CAD build for the part. Positions are in the model's coordinates, mm. A direction names the side the tool comes from. Give positions to 0.01 mm unless a question says otherwise; leave off trailing zeros. Order: outer loops, then holes, each group sorted by start corner. A loop starts at its lowest first (then second) coordinate and runs counter-clockwise, first axis right, second up. Notation, with made-up numbers: (21.5, 37.5) -> (67.5, 37.5) arc R4 cw to (67.5, 43.5) -> close; hole circle Ø5 at (47, 63.5). An arc over 180 degrees is marked (long way). Use one line per item in the form item = value. Start each with the question number.
1) Cut at C-C, the plane x = 31.5. Give the cut face in (y, z), and give its area (3 significant figures).
2) Cut at D-D, the plane y = 24. Give the cut face in (x, z), and give its area (3 significant figures).
3) Cut at B-B, the plane y = 34. Give the cut face in (x, z) (3 decimals), and give its area (3 significant figures).
4) Mould opens along X. For faces 4 (the face through (39, 24, 10)), 5 (the face through (20.75, 19, 3)), 6 (the face through (23.15, 34.5, 1.48)) say: pulls with the +X half, pulls with the -X half, needs draft (parallel to the pull), parting line crosses it, or undercut.
5) Cut at A-A, the plane z = 14. Give the cut face in (x, y).
6) Tool access for faces 1 (the face through (23.18, 6.47, 4.52)), 2 (the face through (35.5, 30, 9)), 3 (the face through (29, 24, 1)): list every direction of +Z, -Z, +X, -X, +Y, -Y with a clear straight run to the whole face (end or side of a thin tool).
7) Probe line 1 (Y direction, x = 30.75, z = 2.7); line 2 (X direction, y = 23, z = 2); line 3 (Y direction, x = 24.75, z = 1.7) (3 decimals). List the from-to ranges inside material, lowest first.
8) Drop flat-ended pins along their axis: P1, Ø4.5, axis at x = 30.75, y = 20, coming from the +Z side; P2, Ø9.5, axis at x = 24.75, y = 34, coming from the -Z side; P3, Ø3, axis at x = 25, y = 4, coming from the +Z side; P4, Ø2, axis at y = 38.5, z = 8, coming from the -X side. Give the stop position or say it passes through.
from build123d import *

# Parameters (mm, degrees)
SKETCH1_W           = 20.75
SKETCH1_H           = 48
SKETCH1_R           = 1.675
BOSS_EXTRUDE1_DEPTH = 6
SKETCH2_W           = 15
SKETCH2_H           = 48
BOSS_EXTRUDE2_DEPTH = 6
SKETCH3_R           = 4
CUT_EXTRUDE1_DEPTH  = 6
SKETCH5_R           = 2.925
CUT_EXTRUDE2_DEPTH  = 3
SKETCH6_R           = 1.75
CUT_EXTRUDE3_DEPTH  = 10
SKETCH7_W           = 3.5
SKETCH7_H           = 8
CUT_EXTRUDE4_DEPTH  = 2.5
SKETCH8_W           = 14.75
SKETCH8_H           = 10
CUT_EXTRUDE5_DEPTH  = 16
SKETCH9_W           = 15
SKETCH9_H           = 48
CUT_EXTRUDE6_DEPTH  = 20.75


with BuildPart() as part:
    # Sketch1 → Boss-Extrude1 (new body)
    with BuildSketch(Plane.XY):
        with Locations((10.375, 24)):
            Rectangle(SKETCH1_W, SKETCH1_H)
        with Locations((16.75, 34)):
            Circle(SKETCH1_R, mode=Mode.SUBTRACT)
        with Locations((16.75, 4)):
            Circle(SKETCH1_R, mode=Mode.SUBTRACT)
    boss_extrude1 = extrude(amount=BOSS_EXTRUDE1_DEPTH)

    # Sketch2 → Boss-Extrude2 (add)
    with BuildSketch(Plane.ZY):
        with Locations((7.5, 24)):
            Rectangle(SKETCH2_W, SKETCH2_H)
    boss_extrude2 = extrude(amount=-BOSS_EXTRUDE2_DEPTH)

    # Sketch3 → Cut-Extrude1 (cut)
    with BuildSketch(Plane.ZY):
        with Locations((14, 24)):
            Circle(SKETCH3_R)
    cut_extrude1 = extrude(amount=-CUT_EXTRUDE1_DEPTH, mode=Mode.SUBTRACT)

    # Sketch5 → Cut-Extrude2 (cut)
    with BuildSketch(Plane.XY.offset(6)):
        with Locations((16.75, 34)):
            Circle(SKETCH5_R)
        with Locations((16.75, 4)):
            Circle(SKETCH5_R)
    cut_extrude2 = extrude(amount=-CUT_EXTRUDE2_DEPTH, mode=Mode.SUBTRACT)

    # Sketch6 → Cut-Extrude3 (cut)
    with BuildSketch(Plane.XY.offset(6)):
        with Locations((10.75, 28)):
            Circle(SKETCH6_R)
        with Locations((17.75, 28)):
            Circle(SKETCH6_R)
        with Locations(Location((10.75, 20, 0), (0, 0, 180))):
            Circle(SKETCH6_R)
        with Locations(Location((17.75, 20, 0), (0, 0, 180))):
            Circle(SKETCH6_R)
    cut_extrude3 = extrude(amount=-CUT_EXTRUDE3_DEPTH, mode=Mode.SUBTRACT)

    # Sketch7 → Cut-Extrude4 (cut)
    with BuildSketch(Plane(origin=(0, 0, 0), x_dir=(-1, 0, 0), z_dir=(0, 0, -1))):
        with Locations((-17.75, 24)):
            Rectangle(SKETCH7_W, SKETCH7_H)
        with Locations((-10.75, 24)):
            Rectangle(SKETCH7_W, SKETCH7_H)
    cut_extrude4 = extrude(amount=-CUT_EXTRUDE4_DEPTH, mode=Mode.SUBTRACT)

    # Sketch8 → Cut-Extrude5 (cut)
    with BuildSketch(Plane.XY.offset(6)):
        with Locations((13.375, 43)):
            Rectangle(SKETCH8_W, SKETCH8_H)
    cut_extrude5 = extrude(amount=-CUT_EXTRUDE5_DEPTH, mode=Mode.SUBTRACT)

    # Mirror3: Boss-Extrude1, Boss-Extrude2, Cut-Extrude1, Cut-Extrude2, Cut-Extrude3, Cut-Extrude4, Cut-Extrude5 across plane
    add(boss_extrude1.mirror(Plane(origin=(20.75, 0, 6), x_dir=(0, 0, 1), z_dir=(-1, 0, 0))))
    add(boss_extrude2.mirror(Plane(origin=(20.75, 0, 6), x_dir=(0, 0, 1), z_dir=(-1, 0, 0))))
    add(cut_extrude1.mirror(Plane(origin=(20.75, 0, 6), x_dir=(0, 0, 1), z_dir=(-1, 0, 0))), mode=Mode.SUBTRACT)
    add(cut_extrude2.mirror(Plane(origin=(20.75, 0, 6), x_dir=(0, 0, 1), z_dir=(-1, 0, 0))), mode=Mode.SUBTRACT)
    add(cut_extrude3.mirror(Plane(origin=(20.75, 0, 6), x_dir=(0, 0, 1), z_dir=(-1, 0, 0))), mode=Mode.SUBTRACT)
    add(cut_extrude4.mirror(Plane(origin=(20.75, 0, 6), x_dir=(0, 0, 1), z_dir=(-1, 0, 0))), mode=Mode.SUBTRACT)
    add(cut_extrude5.mirror(Plane(origin=(20.75, 0, 6), x_dir=(0, 0, 1), z_dir=(-1, 0, 0))), mode=Mode.SUBTRACT)

    # Sketch9 → Cut-Extrude6 (cut)
    with BuildSketch(Plane.ZY):
        with Locations((7.5, 24)):
            Rectangle(SKETCH9_W, SKETCH9_H)
    extrude(amount=-CUT_EXTRUDE6_DEPTH, mode=Mode.SUBTRACT)


solid = part.part
Result:
q1.outline = (0, 0) -> (18.42, 0) -> (18.42, 6) -> (0, 6) -> close; (21.58, 2.5) -> (26.42, 2.5) -> (26.42, 6) -> (21.58, 6) -> close; (29.58, 0) -> (38, 0) -> (38, 6) -> (29.58, 6) -> close
q1.area = 178 mm²
q2.outline = (20.75, 0) -> (22, 0) -> (22, 2.5) -> (25.5, 2.5) -> (25.5, 0) -> (29, 0) -> (29, 2.5) -> (32.5, 2.5) -> (32.5, 0) -> (41.5, 0) -> (41.5, 10) -> (35.5, 10) -> (35.5, 6) -> (20.75, 6) -> close
q2.area = 131 mm²
q3.outline = (20.75, 0) -> (23.075, 0) -> (23.075, 3) -> (21.825, 3) -> (21.825, 6) -> (20.75, 6) -> close; (26.425, 0) -> (41.5, 0) -> (41.5, 15) -> (35.5, 15) -> (35.5, 6) -> (27.675, 6) -> (27.675, 3) -> (26.425, 3) -> close
q3.area = 151 mm²
q4.face_4 = needs draft
q4.face_5 = pulls with the -X half
q4.face_6 = undercut
q5.outline = (35.5, 0) -> (41.5, 0) -> (41.5, 20) -> (35.5, 20) -> close; (35.5, 28) -> (41.5, 28) -> (41.5, 48) -> (35.5, 48) -> close
q6.face_1 = +Z
q6.face_2 = +Z, -X, +Y
q6.face_3 = -Z
q7.line_1 = 0 to 18.25, 21.75 to 26.25, 29.75 to 38
q7.line_2 = 20.75 to 22, 25.5 to 29, 32.5 to 41.5
q7.line_3 = 0 to 2.325, 5.675 to 18.564, 29.436 to 32.325, 35.675 to 38
q8.P1 = 6
q8.P2 = 0
q8.P3 = 3
q8.P4 = 35.5
